from build123d import *

# Parameters (mm, degrees)
SKETCH1_W           = 50
SKETCH1_H           = 10
BOSS_EXTRUDE1_DEPTH = 15
SKETCH3_R           = 4.5
CUT_EXTRUDE1_DEPTH  = 6
SKETCH4_R           = 3
CUT_EXTRUDE2_DEPTH  = 6
CUT_EXTRUDE3_DEPTH  = 30.580398915
CHAMFER1_SIZE       = 2


with BuildPart() as part:
    # Sketch1 → Boss-Extrude1 (new body)
    with BuildSketch(Plane(origin=(0, 0, 0), x_dir=(0, 0, -1), z_dir=(1, 0, 0))):
        Rectangle(SKETCH1_W, SKETCH1_H)
    extrude(amount=BOSS_EXTRUDE1_DEPTH)

    # Sketch3 → Cut-Extrude1 (cut)
    with BuildSketch(Plane(origin=(0, 5, 0), x_dir=(1, 0, 0), z_dir=(0, 1, 0))):
        with Locations(Location((7.5, -18, 0), (0, 0, 270))):
            Circle(SKETCH3_R)
        with Locations(Location((7.5, 18, 0), (0, 0, 270))):
            Circle(SKETCH3_R)
    extrude(amount=-CUT_EXTRUDE1_DEPTH, mode=Mode.SUBTRACT)

    # Sketch4 → Cut-Extrude2 (cut)
    with BuildSketch(Plane(origin=(0, -1, 0), x_dir=(1, 0, 0), z_dir=(0, 1, 0))):
        with Locations(Location((7.5, 18, 0), (0, 0, 270))):
            Circle(SKETCH4_R)
        with Locations(Location((7.5, -18, 0), (0, 0, 270))):
            Circle(SKETCH4_R)
    extrude(amount=-CUT_EXTRUDE2_DEPTH, mode=Mode.SUBTRACT)

    # Sketch5 → Cut-Extrude3 (cut, through all)
    with BuildSketch(Plane(origin=(15, 0, 0), x_dir=(0, 0, -1), z_dir=(1, 0, 0))):
        with BuildLine():
            Line((-4.35, -2), (-10.65, -2))
            ThreePointArc((-10.65, -2), (-10.04440329, -3.857016936), (-8.460468636, -5))
            Line((-8.460468636, -5), (-6.539531364, -5))
            ThreePointArc((-6.539531364, -5), (-4.95559671, -3.857016936), (-4.35, -2))
        make_face()
        with BuildLine():
            ThreePointArc((-4.35, -2), (-7.5, 1.15), (-10.65, -2))
            Line((-10.65, -2), (-4.35, -2))
        make_face()
        with BuildLine():
            Line((-8.460468636, -5), (-10.65, -5))
            Line((-10.65, -5), (-10.65, -9.185427258))
            Line((-10.65, -9.185427258), (-4.35, -9.185427258))
            Line((-4.35, -9.185427258), (-4.35, -5))
            Line((-4.35, -5), (-6.539531364, -5))
            ThreePointArc((-6.539531364, -5), (-7.5, -5.15), (-8.460468636, -5))
        make_face()
        with BuildLine():
            ThreePointArc((-8.460468636, -5), (-10.04440329, -3.857016936), (-10.65, -2))
            Line((-10.65, -2), (-10.65, -5))
            Line((-10.65, -5), (-8.460468636, -5))
        make_face()
        with BuildLine():
            Line((-4.35, -5), (-4.35, -2))
            ThreePointArc((-4.35, -2), (-4.95559671, -3.857016936), (-6.539531364, -5))
            Line((-6.539531364, -5), (-4.35, -5))
        make_face()
        with BuildLine():
            Line((4.35, -2), (4.35, -5))
            Line((4.35, -5), (6.539531364, -5))
            ThreePointArc((6.539531364, -5), (4.95559671, -3.857016936), (4.35, -2))
        make_face()
        with BuildLine():
            Line((10.65, -2), (4.35, -2))
            ThreePointArc((4.35, -2), (4.95559671, -3.857016936), (6.539531364, -5))
            Line((6.539531364, -5), (8.460468636, -5))
            ThreePointArc((8.460468636, -5), (10.04440329, -3.857016936), (10.65, -2))
        make_face()
        with BuildLine():
            ThreePointArc((10.65, -2), (7.5, 1.15), (4.35, -2))
            Line((4.35, -2), (10.65, -2))
        make_face()
        with BuildLine():
            Line((10.65, -5), (10.65, -2))
            ThreePointArc((10.65, -2), (10.04440329, -3.857016936), (8.460468636, -5))
            Line((8.460468636, -5), (10.65, -5))
        make_face()
    extrude(amount=-CUT_EXTRUDE3_DEPTH, mode=Mode.SUBTRACT)

    # Chamfer1
    chamfer1_edges = [part.edges().sort_by_distance(p)[0] for p in [
        (15, 0, 25),
        (15, 0, -25),
        (0, 0, 25),
        (0, 0, -25),
    ]]
    chamfer(chamfer1_edges, length=CHAMFER1_SIZE)


solid = part.part
Could you check a few things on this model? Use its own coordinates, in mm. A direction names the side the tool comes from. Coordinates: 2 decimals unless noted, no trailing zeros. Loops run counter-clockwise (first coordinate to the right, second up) from the corner with the lowest first, then second, coordinate; pieces in that order, holes last. Notation, with made-up numbers: (21, 61) -> (55, 61) arc R18 cw to (55, 82) -> close; hole circle Ø10 at (9, 68.5). An arc over 180 degrees is marked (long way). Answer in a Markdown table with one row per item.
(1) If I drill on probe 1 along Z at (x, y) = (2.5, -4); probe 2 along X at (y, z) = (2.6, 18); probe 3 along X at (y, z) = (-2.75, 18), over which ranges is the centre line in solid material (lowest first)?
Results found:
| item | result |
|---|---|
| probe 1 | z = -25 to -10.65, -4.35 to 4.35, 10.65 to 25 |
| probe 2 | x = 0 to 3, 12 to 15 |
| probe 3 | x = 0 to 4.5, 10.5 to 15 |
(2) Imagine slicing it at C-C (z = 18). List the corners of the cut face in (x, y) for me.
Results found:
| item | result |
|---|---|
| outline | (0, -5) -> (4.5, -5) -> (4.5, -1) -> (3, -1) -> (3, 5) -> (0, 5) -> close; (10.5, -5) -> (15, -5) -> (15, 5) -> (12, 5) -> (12, -1) -> (10.5, -1) -> close |
(3) Imagine slicing it at D-D (x = 13.5). List the corners of the cut face in (y, z) for me.
Results found:
| item | result |
|---|---|
| outline | (-5, -24.5) -> (5, -24.5) -> (5, 24.5) -> (-5, 24.5) -> (-5, 10.65) -> (-2, 10.65) arc R3.15 cw to (-2, 4.35) -> (-5, 4.35) -> (-5, -4.35) -> (-2, -4.35) arc R3.15 cw to (-2, -10.65) -> (-5, -10.65) -> close |
(4) Will these pins go through, and if not, where does the flat tip stop? pin 1 Ø5 at (x, z) = (8.5, -8.5) entering from -Y; pin 2 Ø8 at (x, z) = (7.5, 18) entering from +Y; pin 3 Ø1.5 at (x, z) = (6, -7.5) entering from -Y.
Results found:
| item | result |
|---|---|
| pin 1 | stops at y = -5 |
| pin 2 | stops at y = -1 |
| pin 3 | stops at y = 1.06 |
(5) For faces 1 (the face through (1, 0, 24)), 2 (the face through (9, -1, 21)), 3 (the face through (8, -3, 10.65)), which set-ups out of +Z, -Z, +X, -X, +Y, -Y let a thin tool reach every point of the face, with its end or its side?
Results found:
| item | result |
|---|---|
| face 1 | +Z, -X, +Y, -Y |
| face 2 | +Y |
| face 3 | +X, -X, -Y |
(6) Thinking about a two-plate mould opening in X: for faces 4 (the face through (1, 0, -24)), 5 (the face through (7.698, 2.042, 13.504)), 6 (the face through (7, 0, 25)), which applies, released by +X, released by -X, zero draft, split by the parting line, or undercut?
Results found:
| item | result |
|---|---|
| face 4 | released by -X |
| face 5 | undercut |
| face 6 | zero draft |
(7) Imagine slicing it at A-A (y = -2.5). List the corners of the cut face in (x, z) for me.
Results found:
| item | result |
|---|---|
| outline | (0, -23) -> (2, -25) -> (13, -25) -> (15, -23) -> (15, -10.65) -> (0, -10.65) -> close; (0, -4.35) -> (15, -4.35) -> (15, 4.35) -> (0, 4.35) -> close; (0, 10.65) -> (15, 10.65) -> (15, 23) -> (13, 25) -> (2, 25) -> (0, 23) -> close; hole circle Ø6 at (7.5, -18); hole circle Ø6 at (7.5, 18) |
(8) Imagine slicing it at B-B (x = 7.5). List the corners of the cut face in (y, z) for me, plus the area to 3 significant figures.
Results found:
| item | result |
|---|---|
| outline | (-5, -25) -> (5, -25) -> (5, -22.5) -> (-1, -22.5) -> (-1, -21) -> (-5, -21) -> close; (-5, -15) -> (-1, -15) -> (-1, -13.5) -> (5, -13.5) -> (5, 13.5) -> (-1, 13.5) -> (-1, 15) -> (-5, 15) -> (-5, 10.65) -> (-2, 10.65) arc R3.15 cw to (-2, 4.35) -> (-5, 4.35) -> (-5, -4.35) -> (-2, -4.35) arc R3.15 cw to (-2, -10.65) -> (-5, -10.65) -> close; (-5, 21) -> (-1, 21) -> (-1, 22.5) -> (5, 22.5) -> (5, 25) -> (-5, 25) -> close |
| area | 275 mm^2 |
